Here's how the part is built. I have some questions about the finished solid (model axes, mm). Round coordinates to 2 decimals unless told otherwise and drop trailing zeros. Loops run counter-clockwise (first coordinate to the right, second up) from the corner with the lowest first, then second, coordinate; pieces in that order, holes last. Notation, with made-up numbers: (-10, 74.5) - (2, 74.5) arc R23 ccw to (2, 89.5) - close; hole circle Ø3 at (33.25, 8.25). An arc over 180 degrees is marked (long way). Answer as a JSON object with one key per item and string values. Group by question number.
1) I want a section at A-A, the plane x = 19. Please give me the cut outline in (y, z) (3 decimals).
2) I want a section at D-D, the plane x = 39. Please give me the cut outline in (y, z).
3) Will these pins go through, and if not, where does the flat tip stop? P1, Ø5, axis at x = -38.1, z = 0, coming from the +Y side; P2, Ø1, axis at y = 2.5, z = -3, coming from the +X side; P3, Ø2, axis at y = 1, z = -2, coming from the +X side.
4) I want a section at B-B, the plane y = 1.3. Please give me the cut outline in (x, z) (3 decimals), then the cut area to 3 significant figures.
5) I want a section at C-C, the plane z = 0. Please give me the cut outline in (x, y) (3 decimals).
6) If I drill on line 1 along X through (y, z) = (2.5, 0) (3 decimals); line 2 along Z through (x, y) = (38.1, 1.6) (3 decimals); line 3 along Z through (x, y) = (21.5, 1.55) (3 decimals), over which ranges is the centre line in solid material (lowest first)? Write a range as [from, to].
from build123d import *

# Parameters (mm, degrees)
SKETCH1_R           = 3.175
BOSS_EXTRUDE5_DEPTH = 3.81


with BuildPart() as part:
    # Sketch1 → Boss-Extrude5 (new body)
    with BuildSketch(Plane(origin=(0, 0, 0), x_dir=(1, 0, 0), z_dir=(0, 1, 0))):
        with BuildLine():
            Line((38.1, -7.62), (-38.1, -7.62))
            ThreePointArc((-38.1, -7.62), (-45.72, 0), (-38.1, 7.62))
            Line((-38.1, 7.62), (38.1, 7.62))
            ThreePointArc((38.1, 7.62), (45.72, 0), (38.1, -7.62))
        make_face()
        with Locations(Location((-38.1, 0, 0), (0, 0, 90))):
            Circle(SKETCH1_R, mode=Mode.SUBTRACT)
        with Locations(Location((38.1, 0, 0), (0, 0, 90))):
            Circle(SKETCH1_R, mode=Mode.SUBTRACT)
        with BuildLine():
            Line((-24.266853823, 4.445), (24.266853823, 4.445))
            ThreePointArc((24.266853823, 4.445), (28.711853823, 0), (24.266853823, -4.445))
            Line((24.266853823, -4.445), (-24.266853823, -4.445))
            ThreePointArc((-24.266853823, -4.445), (-28.711853823, 0), (-24.266853823, 4.445))
        make_face(mode=Mode.SUBTRACT)
    extrude(amount=BOSS_EXTRUDE5_DEPTH)


solid = part.part
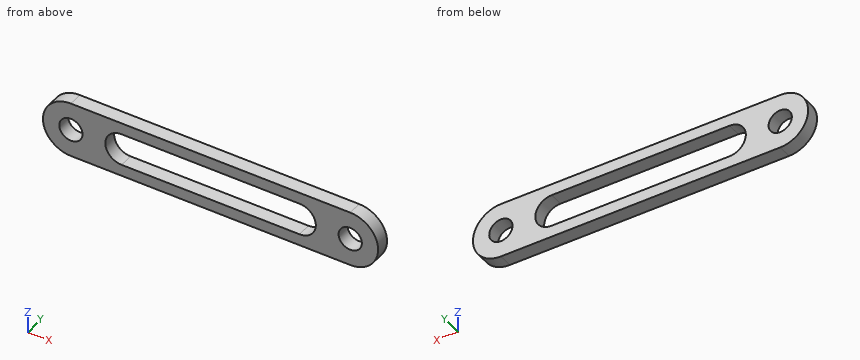
Outcome:
{
 "1": {"outline": "(0, -7.62) - (3.81, -7.62) - (3.81, -4.445) - (0, -4.445) - close; (0, 4.445) - (3.81, 4.445) - (3.81, 7.62) - (0, 7.62) - close"},
 "2": {"outline": "(0, -7.57) - (3.81, -7.57) - (3.81, -3.04) - (0, -3.04) - close; (0, 3.04) - (3.81, 3.04) - (3.81, 7.57) - (0, 7.57) - close"},
 "3": {"P1": "through", "P2": "x = 45.3", "P3": "x = 45.65"},
 "4": {"outline": "(-38.1, -7.62) - (38.1, -7.62) arc R7.62 ccw to (38.1, 7.62) - (-38.1, 7.62) arc R7.62 ccw to start; hole circle Ø6.35 at (-38.1, 0); hole (-24.267, -4.445) - (24.267, -4.445) arc R4.445 ccw to (24.267, 4.445) - (-24.267, 4.445) arc R4.445 ccw to start; hole circle Ø6.35 at (38.1, 0)", "area": "787 mm^2"},
 "5": {"outline": "(-45.72, 0) - (-41.275, 0) - (-41.275, 3.81) - (-45.72, 3.81) - close; (-34.925, 0) - (-28.712, 0) - (-28.712, 3.81) - (-34.925, 3.81) - close; (28.712, 0) - (34.925, 0) - (34.925, 3.81) - (28.712, 3.81) - close; (41.275, 0) - (45.72, 0) - (45.72, 3.81) - (41.275, 3.81) - close"},
 "6": {"line 1": "[-45.72, -41.275], [-34.925, -28.712], [28.712, 34.925], [41.275, 45.72]", "line 2": "[-7.62, -3.175], [3.175, 7.62]", "line 3": "[-7.62, -4.445], [4.445, 7.62]"}
}
